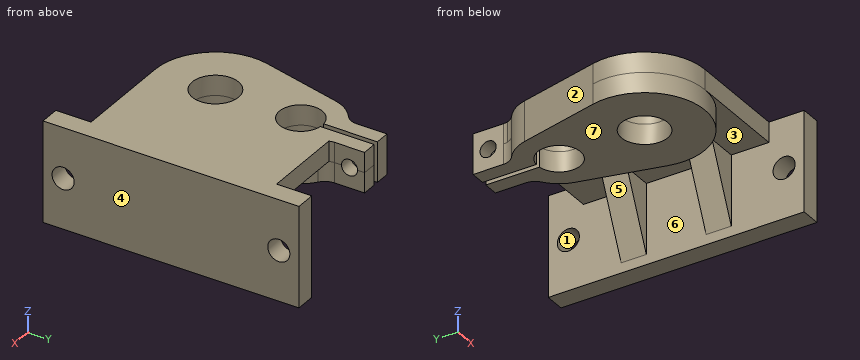
from build123d import *

# Parameters (mm, degrees)
SKETCH_1_R          = 4.6
EXTRUDE_1_DEPTH     = 4
EXTRUDE_START       = -4
SKETCH_1_4_R        = 4.6
EXTRUDE_2_DEPTH     = 4
EXTRUDE_3_DEPTH     = 12
SKETCH_4_R          = 2.2
CUT_EXTRUDE_2_DEPTH = 64.857250973
SKETCH_4_3_R        = 1.6
CUT_EXTRUDE_3_DEPTH = 64.857250973
RIB_6_REACH         = 62.9
SKETCH_6_WALL_W     = 139.031153846
SKETCH_6_WALL_H     = 5
RIB_7_REACH         = 62.9
SKETCH_8_WALL_W     = 139.031153846
SKETCH_8_WALL_H     = 5


with BuildPart() as part:
    # 草图1 → 凸台-拉伸1 (new body)
    with BuildSketch(Plane.XY):
        with BuildLine():
            ThreePointArc((19.272727273, 44.453905218), (17.343879539, 42.438024382), (16.224606286, 39.882352941))
            Line((16.224606286, 39.882352941), (12.336909429, 23.823529412))
            ThreePointArc((12.336909429, 23.823529412), (14.569137024, 13.579836691), (24, 9))
            Line((24, 9), (44, 9))
            Line((44, 9), (44, 2))
            Line((44, 2), (48, 2))
            Line((48, 2), (48, 52.893747285))
            Line((48, 52.893747285), (44, 52.893747285))
            Line((44, 52.893747285), (44, 45.893747285))
            Line((44, 45.893747285), (27.664709895, 45.893747285))
            ThreePointArc((27.664709895, 45.893747285), (27.541464018, 46.377063498), (27.5, 46.874119675))
            Line((27.5, 46.874119675), (27.5, 52.893747285))
            Line((27.5, 52.893747285), (24.5, 52.893747285))
            Line((24.5, 52.893747285), (24.5, 42.220485754))
            ThreePointArc((24.5, 42.220485754), (24, 33.75), (23.5, 42.220485754))
            Line((23.5, 42.220485754), (23.5, 52.893747285))
            Line((23.5, 52.893747285), (20.5, 52.893747285))
            Line((20.5, 52.893747285), (20.5, 46.874119675))
            ThreePointArc((20.5, 46.874119675), (20.458535982, 46.377063498), (20.335290105, 45.893747285))
            ThreePointArc((20.335290105, 45.893747285), (19.913864605, 45.092755684), (19.272727273, 44.453905218))
        make_face()
        with Locations((24, 21)):
            Circle(SKETCH_1_R, mode=Mode.SUBTRACT)
    extrude(amount=EXTRUDE_1_DEPTH)

    # 草图1<4> → 凸台-拉伸2 (add)
    # profile 1 of 2: a face of its own
    with BuildSketch(Plane.XY.offset(EXTRUDE_START)):
        Polygon((44, 45.893747285), (44, 52.893747285), (48, 52.893747285), (48, 2), (44, 2), (44, 9), align=None)
    # profile 2 of 2: a face of its own
    with BuildSketch(Plane.XY.offset(EXTRUDE_START)):
        with BuildLine():
            ThreePointArc((27.5, 46.874119675), (27.824352245, 45.517318624), (28.727272727, 44.453905218))
            ThreePointArc((28.727272727, 44.453905218), (30.656120461, 42.438024382), (31.775393714, 39.882352941))
            Line((31.775393714, 39.882352941), (35.663090571, 23.823529412))
            ThreePointArc((35.663090571, 23.823529412), (24, 9), (12.336909429, 23.823529412))
            Line((12.336909429, 23.823529412), (16.224606286, 39.882352941))
            ThreePointArc((16.224606286, 39.882352941), (17.343879539, 42.438024382), (19.272727273, 44.453905218))
            ThreePointArc((19.272727273, 44.453905218), (20.175647755, 45.517318624), (20.5, 46.874119675))
            Line((20.5, 46.874119675), (20.5, 52.893747285))
            Line((20.5, 52.893747285), (23.5, 52.893747285))
            Line((23.5, 52.893747285), (23.5, 42.220485754))
            ThreePointArc((23.5, 42.220485754), (24, 33.75), (24.5, 42.220485754))
            Line((24.5, 42.220485754), (24.5, 52.893747285))
            Line((24.5, 52.893747285), (27.5, 52.893747285))
            Line((27.5, 52.893747285), (27.5, 46.874119675))
        make_face()
        with Locations((24, 21)):
            Circle(SKETCH_1_4_R, mode=Mode.SUBTRACT)
    extrude(amount=EXTRUDE_2_DEPTH)

    # 草图1<5> → 凸台-拉伸3 (add)
    with BuildSketch(Plane.XY.offset(EXTRUDE_START)):
        Polygon((44, 45.893747285), (44, 52.893747285), (48, 52.893747285), (48, 2), (44, 2), (44, 9), align=None)
    extrude(amount=-EXTRUDE_3_DEPTH)

    # 草图4 → 切除-拉伸2 (cut, through all)
    with BuildSketch(Plane(origin=(44, 0, 0), x_dir=(0, 0, -1), z_dir=(1, 0, 0))):
        with Locations(Location((6, 6, 0), (0, 0, 180))):
            Circle(SKETCH_4_R)
        with Locations(Location((6, 48.893747285, 0), (0, 0, 180))):
            Circle(SKETCH_4_R)
    extrude(amount=CUT_EXTRUDE_2_DEPTH, mode=Mode.SUBTRACT)

    # 草图4<3> → 切除-拉伸3 (cut, through all)
    with BuildSketch(Plane(origin=(44, 0, 0), x_dir=(0, 0, -1), z_dir=(1, 0, 0))):
        with Locations((0, 49.893747285)):
            Circle(SKETCH_4_3_R)
    extrude(amount=-CUT_EXTRUDE_3_DEPTH, mode=Mode.SUBTRACT)

    # 草图6 wall → 筋6 (add, up to next)
    with BuildSketch(Plane(origin=(41, 19, -7), x_dir=(-0.393919298579, 0, 0.919145030018), z_dir=(-0.919145030018, 0, -0.393919298579)), mode=Mode.PRIVATE) as rib_6_sk1:
        Rectangle(SKETCH_6_WALL_W, SKETCH_6_WALL_H)
    rib_6_tool1 = extrude(rib_6_sk1.sketch, amount=-RIB_6_REACH, mode=Mode.PRIVATE) - part.part
    add(rib_6_tool1.solids().sort_by_distance((41, 19, -7))[0])

    # 草图8 wall → 筋7 (add, up to next)
    with BuildSketch(Plane(origin=(41, 35.893747285, -7), x_dir=(-0.393919298579, 0, 0.919145030018), z_dir=(0.919145030018, 0, 0.393919298579)), mode=Mode.PRIVATE) as rib_7_sk1:
        Rectangle(SKETCH_8_WALL_W, SKETCH_8_WALL_H)
    rib_7_tool1 = extrude(rib_7_sk1.sketch, amount=RIB_7_REACH, mode=Mode.PRIVATE) - part.part
    add(rib_7_tool1.solids().sort_by_distance((41, 35.893747285, -7))[0])


solid = part.part
Geometry: final body of the model. Coordinates: model frame, mm. Face numbers are marked on the shaded views. A direction names the side the tool comes from. Round coordinates to 2 decimals unless told otherwise and drop trailing zeros. Loops run counter-clockwise (first coordinate to the right, second up) from the corner with the lowest first, then second, coordinate; pieces in that order, holes last. Notation, with made-up numbers: M 22.25,-24 L 45.25,-24 A22 cw 45.25,-10 Z; hole C -35.75,20.25 d8. An arc over 180 degrees is marked long. Put each result on its own line as item: value. Start each with the question number.
(1) Section query A-A (y = 6). Return loops of the section in (x, z), then the cut area to 3 significant figures.
(2) Section query B-B (z = 1). Return loops of the section in (x, y).
(3) Contact query for flat-ended pins moving along their axis: pin 1 Ø1.2 at (y, z) = (45.5, 3) entering from -X; pin 2 Ø4 at (x, y) = (21, 41) entering from -Z; pin 3 Ø1.2 at (x, z) = (39, 1) entering from +Y. Output: stop coordinate, or through.
(4) Material intervals for line 1 along Y through (x, z) = (46.25, -6); line 2 along X through (y, z) = (45.5, -2.75); line 3 along X through (y, z) = (25, -0.75), sorted ascending. Write a range as [from, to].
(5) Set-up query: the marked faces 4, 5, 6 and 7. Return all of +Z, -Z, +X, -X, +Y, -Y with unobstructed straight access to the full face (end or side cutting, diameter ignored); none if empty.
(6) Draft query along X for the marked faces 1, 2 and 3. Return one class per face: +X half, -X half, draft (parallel to the pull), parting line (faces both ways), or undercut.
(7) Section query D-D (x = 45.5). Return loops of the section in (y, z).
(8) Section query C-C (z = -2.25). Return loops of the section in (x, y), then the cut area to 3 significant figures.
Findings below:
1. outline: M 44,-16 L 48,-16 L 48,-8.2 L 44,-8.2 Z; M 44,-3.8 L 48,-3.8 L 48,4 L 44,4 Z
1. area: 62.4 mm2
2. outline: M 12.34,23.82 A12 ccw 24,9 L 44,9 L 44,2 L 48,2 L 48,52.89 L 44,52.89 L 44,45.89 L 27.66,45.89 A3 cw 27.5,46.87 L 27.5,48.64 L 24.5,48.64 L 24.5,42.22 A4.25 cw long 23.5,42.22 L 23.5,48.64 L 20.5,48.64 L 20.5,46.87 A3 cw 19.27,44.45 A8 ccw 16.22,39.88 Z; M 20.5,51.14 L 23.5,51.14 L 23.5,52.89 L 20.5,52.89 Z; M 24.5,51.14 L 27.5,51.14 L 27.5,52.89 L 24.5,52.89 Z; hole C 24,21 d9.2
3. pin 1: stops at x = 19.76
3. pin 2: stops at z = -4
3. pin 3: stops at y = 45.89
4. line 1: y = [2, 3.8], [8.2, 46.69], [51.09, 52.89]
4. line 2: x = [20.17, 23.5], [24.5, 27.83], [44, 48]
4. line 3: x = [12.62, 21.73], [26.27, 35.38], [44, 48]
5. face 4: +Z, -Z, +X, +Y, -Y
5. face 5: -Z, +Y, -Y
5. face 6: -Z
5. face 7: -Z, -X, +Y, -Y
6. face 1: draft
6. face 2: -X half
6. face 3: undercut
7. outline: M 2,-16 L 52.89,-16 L 52.89,4 L 2,4 Z; hole C 6,-6 d4.4; hole C 48.89,-6 d4.4
8. outline: M 12.34,23.82 A12 ccw long 35.66,23.82 L 31.78,39.88 A8 ccw 28.73,44.45 A3 cw 27.5,46.87 L 27.5,52.89 L 24.5,52.89 L 24.5,42.22 A4.25 cw long 23.5,42.22 L 23.5,52.89 L 20.5,52.89 L 20.5,46.87 A3 cw 19.27,44.45 A8 ccw 16.22,39.88 Z; M 38.96,16.5 L 44,16.5 L 44,2 L 48,2 L 48,52.89 L 44,52.89 L 44,38.39 L 38.96,38.39 L 38.96,33.39 L 44,33.39 L 44,21.5 L 38.96,21.5 Z; hole C 24,21 d9.2
8. area: 847 mm2
